Input: part model. Units: mm. Frame: model coordinates. A direction names the side the tool comes from. Round coordinates to 2 decimals unless told otherwise and drop trailing zeros. Order: outer loops, then holes, each group sorted by start corner. A loop starts at its lowest first (then second) coordinate and runs counter-clockwise, first axis right, second up.
Item 1: First-contact query: pin 1 (1.5 mm diameter, centred on y = 1, z = 6.5, fed in from -X); pin 2 (1.5 mm diameter, centred on y = -3, z = 8.5, fed in from +X); pin 3 (1 mm diameter, centred on y = 2, z = 11.5, fed in from -X). Flat tips, straight axial feed; report the tip coordinate or a pass-through.
Item 2: Cut plane C-C on y = -3.5. Output: boundary loops of the cut face in (x, z), then the cut area to 3 significant figures.
Item 3: Cut plane A-A on y = 0. Output: boundary loops of the cut face in (x, z), then the cut area to 3 significant figures.
Item 4: Cut plane D-D on x = 15.5. Output: boundary loops of the cut face in (y, z).
Item 5: Reachability of faces 5 (the cylindrical face through (15, 0, 7)), 6 (the flat face through (0, 2.5, 7)), 7 (the flat face through (0, 3, 3)), 8 (the cylindrical face through (-15, 0, 7)) from +Z, -Z, +X, -X, +Y, -Y: full face, straight path, thin tool, end or side. Return the list, or none.
Item 6: Cut plane B-B on x = 0. Output: boundary loops of the cut face in (y, z).
Item 7: Mould query, pull axis Z, two halves, no side actions, for faces 1 (the flat face through (0, 3, 10.5)), 2 (the flat face through (0, -2.5, 7)), 3 (the flat face through (0, -4, 12)), 4 (the flat face through (0, 0, 13.5)). Classes: released by +Z, released by -Z, zero draft, split by the parting line, or undercut.
Item 8: Line query: L1, parallel to Z at x = -1.5, y = -3.25; L2, parallel to X at y = 1.5, z = 9.25; L3, parallel to X at y = -1, z = 9. Output: solid intervals per line, ascending.
```python
from build123d import *

# Parameters (mm, degrees)
BOSS_EXTRUDE1_DEPTH = 3
BOSS_EXTRUDE2_DEPTH = 7.5
SKETCH6_W           = 7
SKETCH6_H           = 7.5
CUT_EXTRUDE1_DEPTH  = 7.5


with BuildPart() as part:
    # Sketch1 → Boss-Extrude1 (new body)
    with BuildSketch(Plane.XY):
        with BuildLine():
            Line((-15, 4), (15, 4))
            ThreePointArc((15, 4), (19, 0), (15, -4))
            Line((15, -4), (-15, -4))
            ThreePointArc((-15, -4), (-19, 0), (-15, 4))
        make_face()
    boss_extrude1 = extrude(amount=BOSS_EXTRUDE1_DEPTH)

    # Sketch4 → Boss-Extrude2 (add)
    with BuildSketch(Plane.XY.offset(3)):
        with BuildLine():
            Line((-12.5, 2.5), (12.5, 2.5))
            ThreePointArc((12.5, 2.5), (15, 0), (12.5, -2.5))
            Line((12.5, -2.5), (-12.5, -2.5))
            ThreePointArc((-12.5, -2.5), (-15, 0), (-12.5, 2.5))
        make_face()
    extrude(amount=BOSS_EXTRUDE2_DEPTH)

    # Mirror1: Boss-Extrude1 across plane
    add(boss_extrude1.mirror(Plane.XY.offset(6.75)))

    # Sketch6 → Cut-Extrude1 (cut)
    with BuildSketch(Plane(origin=(0, 2.5, 0), x_dir=(1, 0, 0), z_dir=(0, 1, 0))):
        with Locations((-9, -6.75)):
            Rectangle(SKETCH6_W, SKETCH6_H)
        with Locations((9, -6.75)):
            Rectangle(SKETCH6_W, SKETCH6_H)
    extrude(amount=-CUT_EXTRUDE1_DEPTH, mode=Mode.SUBTRACT)


solid = part.part
```
From the geometry:
1. pin 1: stops at x = -14.99
1. pin 2: stops at x = 13.59
1. pin 3: stops at x = -18.71
2. outline: (-16.94, 0) - (16.94, 0) - (16.94, 3) - (-16.94, 3) - close; (-16.94, 10.5) - (16.94, 10.5) - (16.94, 13.5) - (-16.94, 13.5) - close
2. area: 203 mm2
3. outline: (-19, 0) - (19, 0) - (19, 3) - (15, 3) - (15, 10.5) - (19, 10.5) - (19, 13.5) - (-19, 13.5) - (-19, 10.5) - (-15, 10.5) - (-15, 3) - (-19, 3) - close; hole (-12.5, 3) - (-5.5, 3) - (-5.5, 10.5) - (-12.5, 10.5) - close; hole (5.5, 3) - (12.5, 3) - (12.5, 10.5) - (5.5, 10.5) - close
3. area: 348 mm2
4. outline: (-3.97, 0) - (3.97, 0) - (3.97, 3) - (-3.97, 3) - close; (-3.97, 10.5) - (3.97, 10.5) - (3.97, 13.5) - (-3.97, 13.5) - close
5. face 5: +X
5. face 6: +X, -X, +Y
5. face 7: none
5. face 8: -X
6. outline: (-4, 0) - (4, 0) - (4, 3) - (2.5, 3) - (2.5, 10.5) - (4, 10.5) - (4, 13.5) - (-4, 13.5) - (-4, 10.5) - (-2.5, 10.5) - (-2.5, 3) - (-4, 3) - close
7. face 1: undercut
7. face 2: undercut
7. face 3: zero draft
7. face 4: released by +Z
8. L1: z = 0 to 3, 10.5 to 13.5
8. L2: x = -14.5 to -12.5, -5.5 to 5.5, 12.5 to 14.5
8. L3: x = -14.79 to -12.5, -5.5 to 5.5, 12.5 to 14.79
